Source: three-view drawing plus pictorial views. Frame: mm from the lowest corner of the part. Round coordinates to 2 decimals unless told otherwise and drop trailing zeros. Loops run counter-clockwise (first coordinate to the right, second up) from the corner with the lowest first, then second, coordinate; pieces in that order, holes last. Notation, with made-up numbers: M -36.75,52 L -24.75,52 A20 ccw -24.75,90 Z; hole C 61.25,80.25 d7. An arc over 180 degrees is marked long. Write each question's results on one line, items separated by ' | '.
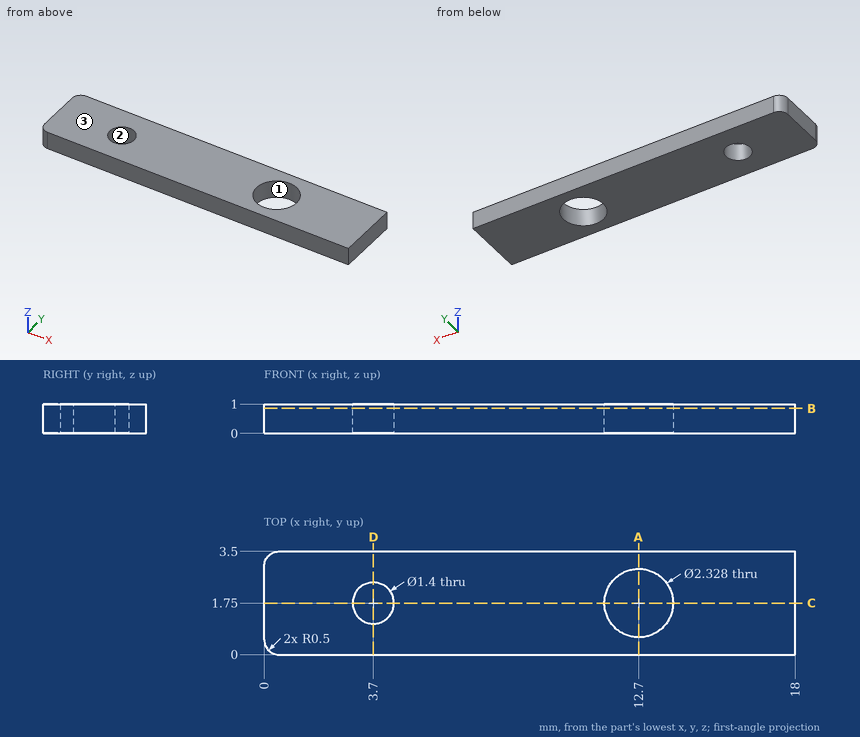
1. Section B-B (z = 0.85). Output: boundary loops of the cut face in (x, y).
Answer key:
outline: M 0,0.5 A0.5 ccw 0.5,0 L 18,0 L 18,3.5 L 0.5,3.5 A0.5 ccw 0,3 Z; hole C 3.7,1.75 d1.4; hole C 12.7,1.75 d2.33
2. Draft query along Y for the marked faces 1, 2 and 3. Return one class per face: pulls with the +Y half, pulls with the -Y half, needs draft (parallel to the pull), parting line crosses it, or undercut.
Answer key:
face 1: undercut | face 2: undercut | face 3: needs draft
3. Section C-C (y = 1.75). Output: boundary loops of the cut face in (x, z), then the cut area to 3 significant figures.
Answer key:
outline: M 0,0 L 3,0 L 3,1 L 0,1 Z; M 4.4,0 L 11.54,0 L 11.54,1 L 4.4,1 Z; M 13.86,0 L 18,0 L 18,1 L 13.86,1 Z | area: 14.3 mm²
4. Pin query (flat end, axial travel): P1, Ø0.8, axis at x = 3.7, y = 1.75, coming from the -Z side. Return the tip coordinate at first contact, or that it passes through.
Answer key:
P1: passes through
5. Ray query, probe 1 along Y at (x, z) = (3.7, 0.5); probe 2 along Y at (x, z) = (12.7, 0.4); probe 3 along X at (y, z) = (2, 0.7). Return the intervals inside material, ascending.
Answer key:
probe 1: y = 0 to 1.05, 2.45 to 3.5 | probe 2: y = 0 to 0.59, 2.91 to 3.5 | probe 3: x = 0 to 3.05, 4.35 to 11.56, 13.84 to 18
6. Section D-D (x = 3.7). Output: boundary loops of the cut face in (y, z), then the cut area to 3 significant figures.
Answer key:
outline: M 0,0 L 1.05,0 L 1.05,1 L 0,1 Z; M 2.45,0 L 3.5,0 L 3.5,1 L 2.45,1 Z | area: 2.10 mm²
7. Section A-A (x = 12.7). Output: boundary loops of the cut face in (y, z), then the cut area to 3 significant figures.
Answer key:
outline: M 0,0 L 0.59,0 L 0.59,1 L 0,1 Z; M 2.91,0 L 3.5,0 L 3.5,1 L 2.91,1 Z | area: 1.17 mm²
